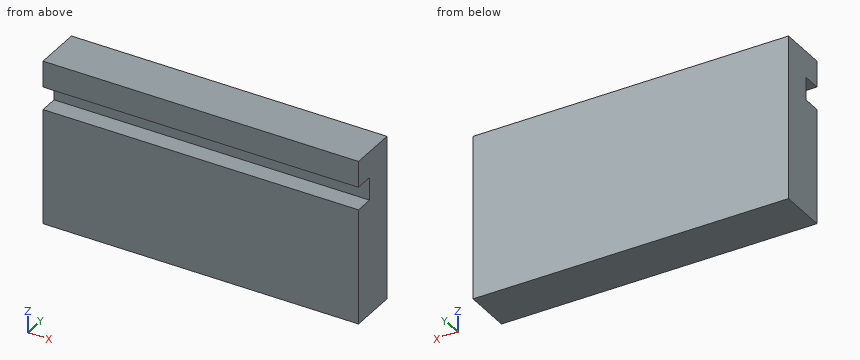
```python
from build123d import *

# Parameters (mm, degrees)
F1_DEPTH      = 120
F1_DEPTH_BACK = 25.4


with BuildPart() as f1:
    # F0 (on Right) → F1 (new body, two sides)
    with BuildSketch(Plane.YZ) as f1_sk:
        Polygon((-21.846049, 0), (0, 0), (0, 75.75617), (-21.846049, 75.75617), (-21.846049, 63.694596), (-13.365726, 63.694596), (-13.365726, 53.186368), (-21.846049, 53.186368), align=None)
    extrude(amount=F1_DEPTH)
    extrude(f1_sk.sketch, amount=-F1_DEPTH_BACK)


solid = f1.part
```
Check sheet for the modelled part. Datum: model origin and axes. Units: mm. Give positions to 0.01 mm unless a question says otherwise; leave off trailing zeros. Write each loop counter-clockwise with the first axis right and the second up, starting at its lowest first coordinate (ties: lowest second). Pieces come first, ordered by that corner, then holes. Notation, with made-up numbers: (43.5, 38.5) - (50.5, 38.5) arc R24 cw to (50.5, 62.5) - close; hole circle Ø1 at (83, 68.25). An arc over 180 degrees is marked (long way). Answer as a JSON object with one key per item and string values. Group by question number.
1) Sectioned sample at A-A (y = -19.5). Record the cut outline in (x, z).
2) Thickness scan on probe 1 along Z at (x, y) = (64, -14); probe 2 along Y at (x, z) = (107, 55). Record the ranges inside material, lowest first. Write a range as from..to.
3) Sectioned sample at B-B (x = 110). Record the cut outline in (y, z).
4) Depth check by flat-ended pin: P1, Ø8.5, axis at x = 29.5, z = 59, coming from the -Y side. Enter the tip coordinate at first touch or a pass-through.
5) Sectioned sample at C-C (z = 61.5). Record the cut outline in (x, y).
Geometry results:
{
 "1": {"outline": "(-25.4, 0) - (120, 0) - (120, 53.19) - (-25.4, 53.19) - close; (-25.4, 63.69) - (120, 63.69) - (120, 75.76) - (-25.4, 75.76) - close"},
 "2": {"probe 1": "z = 0..53.19, 63.69..75.76", "probe 2": "y = -13.37..0"},
 "3": {"outline": "(-21.85, 0) - (0, 0) - (0, 75.76) - (-21.85, 75.76) - (-21.85, 63.69) - (-13.37, 63.69) - (-13.37, 53.19) - (-21.85, 53.19) - close"},
 "4": {"P1": "stops at y = -13.37"},
 "5": {"outline": "(-25.4, -13.37) - (120, -13.37) - (120, 0) - (-25.4, 0) - close"}
}
